from build123d import *

# Parameters (mm, degrees)
ESQUISSE1_W                                = 17.7
ESQUISSE1_H                                = 17.95
BOSS_EXTRU_1_DEPTH                         = 8
ENL_V_MAT_EXTRU_1_DEPTH                    = 8
SYM_TRIE1_AT_THE_SECOND_PLANE_COPY_1_DEPTH = 8
ESQUISSE4_R                                = 7.334991569
BOSS_EXTRU_2_DEPTH                         = 1.5
ESQUISSE5_R                                = 1.475
BOSS_EXTRU_3_DEPTH                         = 3
ESQUISSE6_R                                = 6.208536563
BOSS_EXTRU_4_DEPTH                         = 1
ESQUISSE7_W                                = 25.4
ESQUISSE7_H                                = 26.6
BOSS_EXTRU_5_DEPTH                         = 1.7
CONG_1_R                                   = 1
CONG_2_R                                   = 1
ESQUISSE8_R                                = 0.384895333
ENL_V_MAT_EXTRU_2_DEPTH                    = 1.7
SYM_TRIE5_AT_THE_SECOND_PLANE_COPY_1_SKE_R = 0.384895333
SYM_TRIE5_AT_THE_SECOND_PLANE_COPY_1_DEPTH = 1.7


with BuildPart() as part:
    # Esquisse1 → Boss.-Extru.1 (new body)
    with BuildSketch(Plane(origin=(0, 0, 0), x_dir=(1, 0, 0), z_dir=(0, 1, 0))):
        Rectangle(ESQUISSE1_W, ESQUISSE1_H)
    extrude(amount=BOSS_EXTRU_1_DEPTH)

    # Esquisse2 → Enlèv. mat.-Extru.1 (cut)
    with BuildSketch(Plane(origin=(0, 8, 0), x_dir=(1, 0, 0), z_dir=(0, 1, 0))):
        Polygon((-8.85, -6.975), (-6.85, -8.975), (-8.85, -8.975), align=None)
    enl_v_mat_extru_1 = extrude(amount=-ENL_V_MAT_EXTRU_1_DEPTH, mode=Mode.SUBTRACT)

    # Symétrie1: Enlèv. mat.-Extru.1 across plane
    add(enl_v_mat_extru_1.mirror(Plane.XY), mode=Mode.SUBTRACT)

    # Symétrie1 at the second plane: Enlèv. mat.-Extru.1 across plane
    add(enl_v_mat_extru_1.mirror(Plane(origin=(0, 0, 0), x_dir=(0, 0, 1), z_dir=(1, 0, 0))), mode=Mode.SUBTRACT)

    # Symétrie1 at the second plane copy 1 ske → Symétrie1 at the second plane copy 1 (cut)
    with BuildSketch(Plane(origin=(0, 8, 0), x_dir=(-1, 0, 0), z_dir=(0, 1, 0))):
        Polygon((-8.85, -6.975), (-6.85, -8.975), (-8.85, -8.975), align=None)
    extrude(amount=-SYM_TRIE1_AT_THE_SECOND_PLANE_COPY_1_DEPTH, mode=Mode.SUBTRACT)

    # Esquisse4 → Boss.-Extru.2 (add)
    with BuildSketch(Plane(origin=(0, 8, 0), x_dir=(1, 0, 0), z_dir=(0, 1, 0))):
        with Locations(Location((0, 0, 0), (0, 0, 270))):
            Circle(ESQUISSE4_R)
    extrude(amount=BOSS_EXTRU_2_DEPTH)

    # Esquisse5 → Boss.-Extru.3 (add)
    with BuildSketch(Plane(origin=(0, 9.5, 0), x_dir=(1, 0, 0), z_dir=(0, 1, 0))):
        with Locations(Location((0, 0, 0), (0, 0, 270))):
            Circle(ESQUISSE5_R)
    extrude(amount=BOSS_EXTRU_3_DEPTH)

    # Esquisse6 → Boss.-Extru.4 (add)
    with BuildSketch(Plane(origin=(0, 12.5, 0), x_dir=(1, 0, 0), z_dir=(0, 1, 0))):
        with Locations(Location((0, 0, 0), (0, 0, 270))):
            Circle(ESQUISSE6_R)
    extrude(amount=BOSS_EXTRU_4_DEPTH)

    # Esquisse7 → Boss.-Extru.5 (add)
    with BuildSketch(Plane.XZ):
        Rectangle(ESQUISSE7_W, ESQUISSE7_H)
    extrude(amount=BOSS_EXTRU_5_DEPTH)

    # Congé1
    cong_1_edges = [part.edges().sort_by_distance(p)[0] for p in [
        (12.7, -0.85, 13.3),
    ]]
    fillet(cong_1_edges, radius=CONG_1_R)

    # Congé2
    cong_2_edges = [part.edges().sort_by_distance(p)[0] for p in [
        (12.7, -0.85, -13.3),
        (-12.7, -0.85, 13.3),
        (-12.7, -0.85, -13.3),
    ]]
    fillet(cong_2_edges, radius=CONG_2_R)

    # Esquisse8 → Enlèv. mat.-Extru.2 (cut)
    with BuildSketch(Plane.XZ.offset(1.7)):
        with Locations(Location((-11.7, -12.3, 0), (0, 0, 270))):
            Circle(ESQUISSE8_R)
    enl_v_mat_extru_2 = extrude(amount=-ENL_V_MAT_EXTRU_2_DEPTH, mode=Mode.SUBTRACT)

    # Symétrie5: Enlèv. mat.-Extru.2 across plane
    add(enl_v_mat_extru_2.mirror(Plane.XY), mode=Mode.SUBTRACT)

    # Symétrie5 at the second plane: Enlèv. mat.-Extru.2 across plane
    add(enl_v_mat_extru_2.mirror(Plane(origin=(0, 0, 0), x_dir=(0, 0, 1), z_dir=(1, 0, 0))), mode=Mode.SUBTRACT)

    # Symétrie5 at the second plane copy 1 ske → Symétrie5 at the second plane copy 1 (cut)
    with BuildSketch(Plane(origin=(0, -1.7, 0), x_dir=(-1, 0, 0), z_dir=(0, -1, 0))):
        with Locations(Location((-11.7, -12.3, 0), (0, 0, 270))):
            Circle(SYM_TRIE5_AT_THE_SECOND_PLANE_COPY_1_SKE_R)
    extrude(amount=-SYM_TRIE5_AT_THE_SECOND_PLANE_COPY_1_DEPTH, mode=Mode.SUBTRACT)


solid = part.part
CAD build for the part. Positions are in the model's coordinates, mm. A direction names the side the tool comes from. Round coordinates to 2 decimals unless told otherwise and drop trailing zeros. Loops run counter-clockwise (first coordinate to the right, second up) from the corner with the lowest first, then second, coordinate; pieces in that order, holes last. Notation, with made-up numbers: M 64,-38 L 119,-38 A20 ccw 119,-27 Z; hole C -9,87.5 d1. An arc over 180 degrees is marked long. One line per question, with ' | ' between items. Start each with the question number.
Item 1: Cut at A-A, the plane x = -3. Write the cut outline in (y, z) (3 decimals).
Item 2: Cut at C-C, the plane y = 5. Write the cut outline in (x, z) (3 decimals).
Item 3: Cut at B-B, the plane z = 2. Write the cut outline in (x, y), plus the area to 3 significant figures.
Item 4: Pin check, flat tips, straight feed: pin 1 Ø1.5 at (y, z) = (5, -3.5) entering from +X; pin 2 Ø6 at (y, z) = (9.5, -1) entering from -X. Stop position of each tip, or through.
Item 5: Two-plate mould, pull along Y, no slides. Class faces 1 (the flat face through (-7.864, 4.056, -7.961)), 2 (the flat face through (0, 9.5, 2)), 3 (the flat face through (0, 0, 12)): pulls with the +Y half, pulls with the -Y half, needs draft (parallel to the pull), parting line crosses it, or undercut.
Item 6: Which spindle directions (+Z, -Z, +X, -X, +Y, -Y) get a long thin tool onto all of the face, cutting with end or side? Do faces 4 (the flat face through (-8.85, 4, 0)), 5 (the flat face through (0, 4, -8.975)), 6 (the flat face through (7.864, 4.056, -7.961)), 7 (the cylindrical face through (-7.16, 8.74, -1.59)), 8 (the flat face through (0, 4, 8.975)). Say none if no direction does.
Item 7: Cut at D-D, the plane z = -11.5. Write the cut outline in (x, y).
Item 8: Wall check: line 1 (X direction, y = -0.35, z = 12.3); line 2 (Z direction, x = 11.7, y = -1.15); line 3 (Y direction, x = -3.25, z = 0.25). Give the ranges that are in metal, low to high.
Responses:
1) outline: M -1.7,-13.3 L 0,-13.3 L 0,-8.975 L 8,-8.975 L 8,-6.693 L 9.5,-6.693 L 9.5,6.693 L 8,6.693 L 8,8.975 L 0,8.975 L 0,13.3 L -1.7,13.3 Z; M 12.5,-5.436 L 13.5,-5.436 L 13.5,5.436 L 12.5,5.436 Z
2) outline: M -8.85,-6.975 L -6.85,-8.975 L 6.85,-8.975 L 8.85,-6.975 L 8.85,6.975 L 6.85,8.975 L -6.85,8.975 L -8.85,6.975 Z
3) outline: M -12.7,-1.7 L 12.7,-1.7 L 12.7,0 L 8.85,0 L 8.85,8 L 7.06,8 L 7.06,9.5 L -7.06,9.5 L -7.06,8 L -8.85,8 L -8.85,0 L -12.7,0 Z; M -5.88,12.5 L 5.88,12.5 L 5.88,13.5 L -5.88,13.5 Z | area: 218 mm²
4) pin 1: stops at x = 8.85 | pin 2: stops at x = -8.85
5) face 1: needs draft | face 2: undercut | face 3: pulls with the +Y half
6) face 4: +Z, -Z, -X, +Y | face 5: -Z, +X, -X, +Y | face 6: -Z, +X, +Y | face 7: +Y | face 8: +Z, +X, -X, +Y
7) outline: M -12.7,-1.7 L 12.7,-1.7 L 12.7,0 L -12.7,0 Z
8) line 1: x = -12.7 to -12.08, -11.32 to 11.32, 12.08 to 12.7 | line 2: z = -13.3 to -12.68, -11.92 to 11.92, 12.68 to 13.3 | line 3: y = -1.7 to 9.5, 12.5 to 13.5
